Can you work these out from the model? Positions are in its coordinate system, mm. Round coordinates to 2 decimals unless told otherwise and drop trailing zeros. Loops run counter-clockwise (first coordinate to the right, second up) from the corner with the lowest first, then second, coordinate; pieces in that order, holes last. Notation, with made-up numbers: (19.25, -1) -> (45.25, -1) arc R30 ccw to (45.25, 22) -> close; hole circle Ø6 at (53.25, 47). An arc over 180 degrees is marked (long way). Write item = value, one per line.
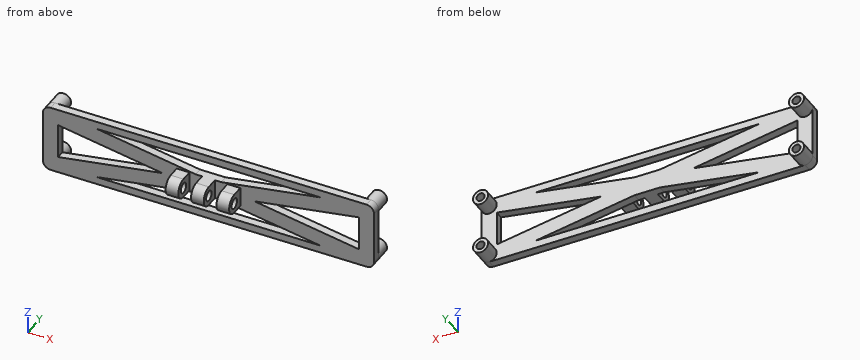
from build123d import *

# Parameters (mm, degrees)
BOSS_EXTRUDE2_DEPTH = 2
SKETCH4_R           = 1.835
BOSS_EXTRUDE3_DEPTH = 4
SKETCH6_R           = 0.985
CUT_EXTRUDE1_DEPTH  = 4
SKETCH7_R           = 1.25
BOSS_EXTRUDE4_DEPTH = 3.086
SKETCH8_R           = 1.25
BOSS_EXTRUDE5_DEPTH = 1.543
BOSS_EXTRUDE6_START = 3.086
SKETCH9_R           = 1.25
BOSS_EXTRUDE6_DEPTH = 3.086


with BuildPart() as part:
    # Sketch3 → Boss-Extrude2 (new body)
    with BuildSketch(Plane(origin=(0, 0, 0), x_dir=(1, 0, 0), z_dir=(0, 1, 0))):
        with BuildLine():
            Line((38.36, -8.225), (-38.36, -8.225))
            ThreePointArc((-38.36, -8.225), (-39.657541, -7.687541), (-40.195, -6.39))
            Line((-40.195, -6.39), (-40.195, 6.39))
            ThreePointArc((-40.195, 6.39), (-39.657541, 7.687541), (-38.36, 8.225))
            Line((-38.36, 8.225), (38.36, 8.225))
            ThreePointArc((38.36, 8.225), (39.657541, 7.687541), (40.195, 6.39))
            Line((40.195, 6.39), (40.195, -6.39))
            ThreePointArc((40.195, -6.39), (39.657541, -7.687541), (38.36, -8.225))
        make_face()
        Polygon((-3.089899, 2.375), (3.089899, 2.375), (27.192466, 6.39), (-27.192466, 6.39), align=None, mode=Mode.SUBTRACT)
        Polygon((3.089899, -2.375), (27.192466, -6.39), (-27.192466, -6.39), (-3.089899, -2.375), align=None, mode=Mode.SUBTRACT)
        Polygon((-36.525, 4.224041), (-36.525, -4.224041), (-11.167534, 0), align=None, mode=Mode.SUBTRACT)
        Polygon((36.525, -4.224041), (11.167534, 0), (36.525, 4.224041), align=None, mode=Mode.SUBTRACT)
    extrude(amount=BOSS_EXTRUDE2_DEPTH)

    # Sketch4 → Boss-Extrude3 (add)
    with BuildSketch(Plane(origin=(0, 2, 0), x_dir=(1, 0, 0), z_dir=(0, 1, 0))):
        with Locations(Location((-38.36, 6.39, 0), (0, 0, 90))):
            Circle(SKETCH4_R)
        with Locations(Location((-38.36, -6.39, 0), (0, 0, 270))):
            Circle(SKETCH4_R)
        with Locations(Location((38.36, 6.39, 0), (0, 0, 90))):
            Circle(SKETCH4_R)
        with Locations(Location((38.36, -6.39, 0), (0, 0, 270))):
            Circle(SKETCH4_R)
    extrude(amount=BOSS_EXTRUDE3_DEPTH)

    # Sketch6 → Cut-Extrude1 (cut)
    with BuildSketch(Plane(origin=(0, 6, 0), x_dir=(1, 0, 0), z_dir=(0, 1, 0))):
        with Locations(Location((-38.36, 6.39, 0), (0, 0, 270))):
            Circle(SKETCH6_R)
        with Locations(Location((-38.36, -6.39, 0), (0, 0, 270))):
            Circle(SKETCH6_R)
        with Locations(Location((38.36, 6.39, 0), (0, 0, 270))):
            Circle(SKETCH6_R)
        with Locations(Location((38.36, -6.39, 0), (0, 0, 270))):
            Circle(SKETCH6_R)
    extrude(amount=-CUT_EXTRUDE1_DEPTH, mode=Mode.SUBTRACT)

    # Sketch7 → Boss-Extrude4 (add)
    with BuildSketch(Plane.ZY.offset(-7.715)):
        with BuildLine():
            Line((2.375, -2.775), (2.375, 0))
            Line((2.375, 0), (-2.375, 0))
            Line((-2.375, 0), (-2.375, -2.775))
            ThreePointArc((-2.375, -2.775), (0, -5.15), (2.375, -2.775))
        make_face()
        with Locations((0, -2.775)):
            Circle(SKETCH7_R, mode=Mode.SUBTRACT)
    extrude(amount=BOSS_EXTRUDE4_DEPTH)

    # Sketch8 → Boss-Extrude5 (add, symmetric)
    with BuildSketch(Plane.ZY):
        with BuildLine():
            Line((2.375, 0), (-2.375, 0))
            Line((-2.375, 0), (-2.375, -2.775))
            ThreePointArc((-2.375, -2.775), (0, -5.15), (2.375, -2.775))
            Line((2.375, -2.775), (2.375, 0))
        make_face()
        with Locations((0, -2.775)):
            Circle(SKETCH8_R, mode=Mode.SUBTRACT)
    extrude(amount=BOSS_EXTRUDE5_DEPTH, both=True)

    # Sketch9 → Boss-Extrude6 (add)
    with BuildSketch(Plane(origin=(-7.715, 0, 0), x_dir=(0, 0, 1), z_dir=(1, 0, 0)).offset(BOSS_EXTRUDE6_START)):
        with BuildLine():
            Line((-2.375, 0), (2.375, 0))
            Line((2.375, 0), (2.375, 2.775))
            ThreePointArc((2.375, 2.775), (0, 5.15), (-2.375, 2.775))
            Line((-2.375, 2.775), (-2.375, 0))
        make_face()
        with Locations((0, 2.775)):
            Circle(SKETCH9_R, mode=Mode.SUBTRACT)
    extrude(amount=-BOSS_EXTRUDE6_DEPTH)


solid = part.part
1. I'm going to push flat-ended pins straight in: pin 1 (1.8 mm diameter, centred on x = -38.36, z = 6.39, fed in from -Y); pin 2 (4 mm diameter, centred on y = -2.5, z = 0.5, fed in from -X) (3 decimals); pin 3 (3 mm diameter, centred on x = 9.5, y = -3.5, fed in from +Z); pin 4 (1.6 mm diameter, centred on x = -38.36, z = -6.39, fed in from +Y). Where does each tip first touch, or does it pass through?
Entries:
pin_1 = 0
pin_2 = -7.715
pin_3 = through
pin_4 = 2
2. I need wall thicknesses on line 1 (X direction, y = 3.1, z = -6.39) (3 decimals); line 2 (Z direction, x = -3, y = 0.5) (3 decimals); line 3 (Y direction, x = 2, z = 1). Which ranges of each line are inside material? Lowest first, please. Write a range as [from, to].
Entries:
line_1 = [-40.195, -39.345], [-37.375, -36.525], [36.525, 37.375], [39.345, 40.195]
line_2 = [-8.225, -6.39], [-2.375, 2.375], [6.39, 8.225]
line_3 = [0, 2]
3. Suppose I cut it at D-D, the plane z = -3.25. List the corners of the cut face in (x, y) for me (3 decimals).
Entries:
outline = (-40.195, 0) -> (-36.525, 0) -> (-36.525, 2) -> (-40.195, 2) -> close; (-30.678, 0) -> (-8.343, 0) -> (-8.343, 2) -> (-30.678, 2) -> close; (8.343, 0) -> (30.678, 0) -> (30.678, 2) -> (8.343, 2) -> close; (36.525, 0) -> (40.195, 0) -> (40.195, 2) -> (36.525, 2) -> close
4. Suppose I cut it at C-C, the plane x = 22. List the corners of the cut face in (y, z) for me (3 decimals).
Entries:
outline = (0, -8.225) -> (2, -8.225) -> (2, -6.39) -> (0, -6.39) -> close; (0, -5.525) -> (2, -5.525) -> (2, -1.804) -> (0, -1.804) -> close; (0, 1.804) -> (2, 1.804) -> (2, 5.525) -> (0, 5.525) -> close; (0, 6.39) -> (2, 6.39) -> (2, 8.225) -> (0, 8.225) -> close
5. Suppose I cut it at A-A, the plane y = 4. List the corners of the cut face in (x, z) for me (3 decimals).
Entries:
outline = circle Ø3.67 at (-38.36, -6.39); circle Ø3.67 at (-38.36, 6.39); circle Ø3.67 at (38.36, -6.39); circle Ø3.67 at (38.36, 6.39); hole circle Ø1.97 at (-38.36, -6.39); hole circle Ø1.97 at (-38.36, 6.39); hole circle Ø1.97 at (38.36, -6.39); hole circle Ø1.97 at (38.36, 6.39)
6. Suppose I cut it at B-B, the plane y = 1. List the corners of the cut face in (x, z) for me (3 decimals), and give its area (3 significant figures).
Entries:
outline = (-40.195, -6.39) arc R1.835 ccw to (-38.36, -8.225) -> (38.36, -8.225) arc R1.835 ccw to (40.195, -6.39) -> (40.195, 6.39) arc R1.835 ccw to (38.36, 8.225) -> (-38.36, 8.225) arc R1.835 ccw to (-40.195, 6.39) -> close; hole (-36.525, -4.224) -> (-11.168, 0) -> (-36.525, 4.224) -> close; hole (-27.192, -6.39) -> (27.192, -6.39) -> (3.09, -2.375) -> (-3.09, -2.375) -> close; hole (-27.192, 6.39) -> (-3.09, 2.375) -> (3.09, 2.375) -> (27.192, 6.39) -> close; hole (11.168, 0) -> (36.525, -4.224) -> (36.525, 4.224) -> close
area = 862 mm²
